Autodesk Fusion 360 part; units mm, degrees
sketch "Sketch1" plane through (0, 0, 0) normal (0, 1, 0) x (1, 0, 0)
  line L0 (28, 6.5) -> (-28, 6.5)
  line L1 (-30, 4.5) -> (-30, -4.5)
  line L2 (-28, -6.5) -> (28, -6.5)
  line L3 (30, -4.5) -> (30, 4.5)
  line L4 (30, 6.5) -> (-30, -6.5) construction
  line L5 (-30, 6.5) -> (30, -6.5) construction
  arc A0 (-30, -4.5) -> (-28, -6.5) centre (-28, -4.5) ccw
  arc A1 (28, -6.5) -> (30, -4.5) centre (28, -4.5) ccw
  arc A2 (30, 4.5) -> (28, 6.5) centre (28, 4.5) ccw
  arc A3 (-28, 6.5) -> (-30, 4.5) centre (-28, 4.5) ccw
  line L6 (0, 0) -> (20, 0) construction
  line L7 (0, 0) -> (-20, 0) construction
  circle A4 centre (20, 0) radius 3
  circle A5 centre (-20, 0) radius 3
  dimension "d1" = 60
  dimension "d2" = 13
  dimension "d3" = 2
  dimension "d4" = 2
  dimension "d5" = 20
  dimension "d6" = 20
  dimension "d7" = 6
  dimension "d8" = 6
extrude "Extrude1" add sketch "Sketch1" along normal blind 3
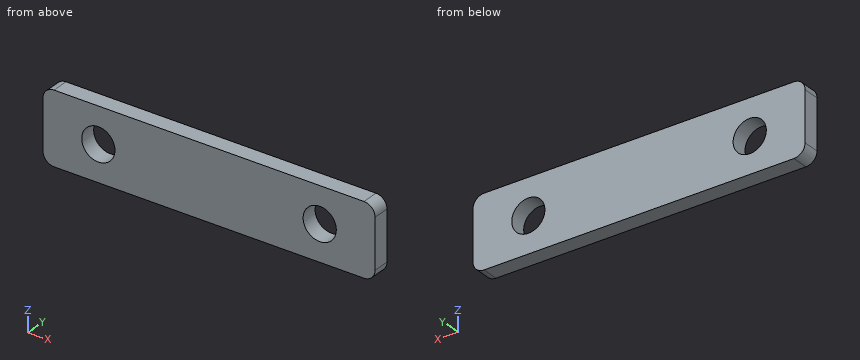
CAD build for the part. Positions are in the model's coordinates, mm. Coordinates: 2 decimals unless noted, no trailing zeros. Write each loop counter-clockwise with the first axis right and the second up, starting at its lowest first coordinate (ties: lowest second). Pieces come first, ordered by that corner, then holes. Notation, with made-up numbers: M 29,41.5 L 77,41.5 A31 ccw 77,66.5 Z; hole C -7,20.5 d6. An arc over 180 degrees is marked long. Answer as a JSON object with one key per item and string values. Group by question number.
1) Saw through at A-A (z = 0). Write the cut outline in (x, y), plus the area to 3 significant figures.
2) Wall check: line 1 (X direction, y = 1.95, z = 0); line 2 (Z direction, x = -20, y = 1.25); line 3 (X direction, y = 2.75, z = -2). Give the ranges that are in metal, low to high. Write a range as from..to.
3) Pin check, flat tip, straight feed: pin 1 Ø5.5 at (x, z) = (20, 0) entering from +Y. Stop position of the tip, or through.
4) Saw through at C-C (x = 20). Write the cut outline in (y, z), plus the area to 3 significant figures.
5) Saw through at B-B (y = 0.45). Write the cut outline in (x, z), plus the area to 3 significant figures.
6) Saw through at D-D (x = -19.5). Write the cut outline in (y, z).
Values follow:
{
 "1": {"outline": "M -30,0 L -23,0 L -23,3 L -30,3 Z; M -17,0 L 17,0 L 17,3 L -17,3 Z; M 23,0 L 30,0 L 30,3 L 23,3 Z", "area": "144 mm2"},
 "2": {"line 1": "x = -30..-23, -17..17, 23..30", "line 2": "z = -6.5..-3, 3..6.5", "line 3": "x = -30..-22.24, -17.76..17.76, 22.24..30"},
 "3": {"pin 1": "passes through"},
 "4": {"outline": "M 0,-6.5 L 3,-6.5 L 3,-3 L 0,-3 Z; M 0,3 L 3,3 L 3,6.5 L 0,6.5 Z", "area": "21.0 mm2"},
 "5": {"outline": "M -30,-4.5 A2 ccw -28,-6.5 L 28,-6.5 A2 ccw 30,-4.5 L 30,4.5 A2 ccw 28,6.5 L -28,6.5 A2 ccw -30,4.5 Z; hole C -20,0 d6; hole C 20,0 d6", "area": "720 mm2"},
 "6": {"outline": "M 0,-6.5 L 3,-6.5 L 3,-2.96 L 0,-2.96 Z; M 0,2.96 L 3,2.96 L 3,6.5 L 0,6.5 Z"}
}
